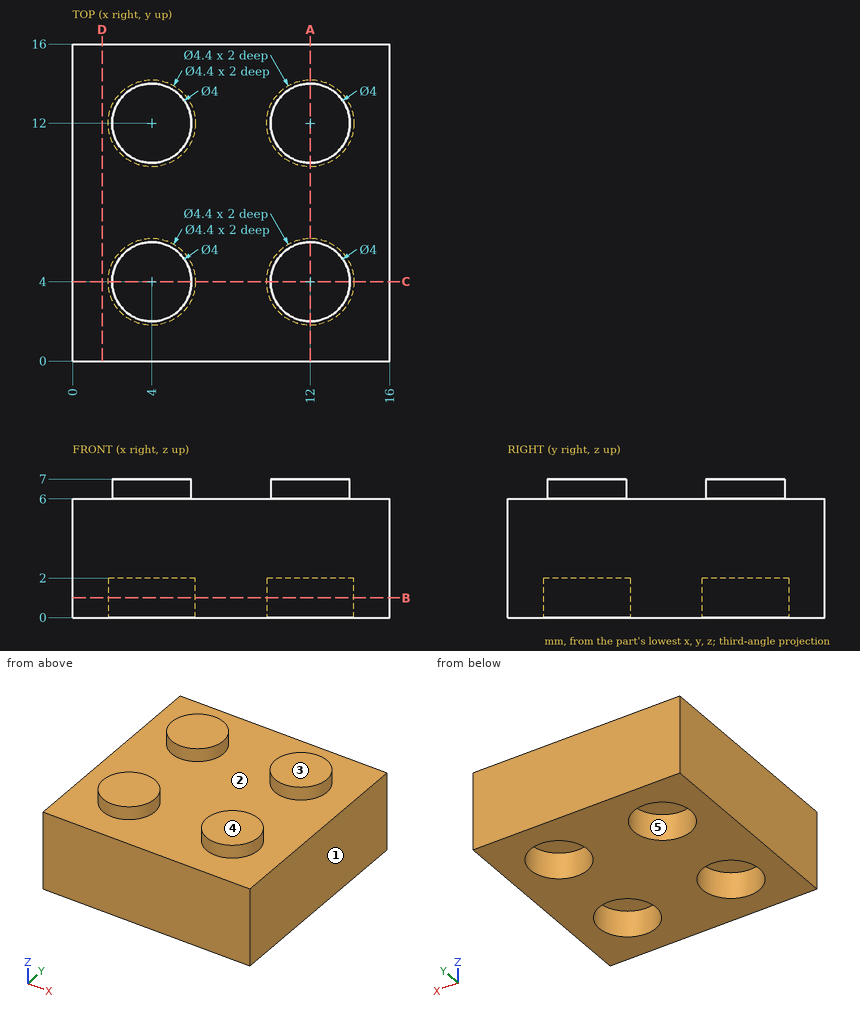
Input: dimensioned drawing with shaded views. Units: mm. Origin: part minimum x, y, z. A direction names the side the tool comes from. Coordinates: 2 decimals unless noted, no trailing zeros. Loops run counter-clockwise (first coordinate to the right, second up) from the corner with the lowest first, then second, coordinate; pieces in that order, holes last. Notation, with made-up numbers: M -30.5,-22.5 L -24.5,-22.5 A32 cw -24.5,14.5 Z; hole C 1,88 d9. An arc over 180 degrees is marked long. One line per item, written item: value.
(1) Section B-B (z = 1). Output: boundary loops of the cut face in (x, y).
Filled in:
outline: M 0,0 L 16,0 L 16,16 L 0,16 Z; hole C 4,4 d4.4; hole C 4,12 d4.4; hole C 12,4 d4.4; hole C 12,12 d4.4
(2) Section A-A (x = 12). Output: boundary loops of the cut face in (y, z), and give its area (3 significant figures).
Filled in:
outline: M 0,0 L 1.8,0 L 1.8,2 L 6.2,2 L 6.2,0 L 9.8,0 L 9.8,2 L 14.2,2 L 14.2,0 L 16,0 L 16,6 L 14,6 L 14,7 L 10,7 L 10,6 L 6,6 L 6,7 L 2,7 L 2,6 L 0,6 Z
area: 86.4 mm^2
(3) Pin query (flat end, axial travel): pin 1 (2.5 mm diameter, centred on x = 12, y = 12, fed in from -Z). Return the tip coordinate at first contact, or that it passes through.
Filled in:
pin 1: z = 2
(4) Pull-direction query (X, two-part tool) for the marked faces 1, 2 and 3; classes: +X half, -X half, draft (parallel to the pull), parting line (faces both ways), or undercut.
Filled in:
face 1: +X half
face 2: undercut
face 3: draft
(5) Reachability of the marked faces 4 and 5 from +Z, -Z, +X, -X, +Y, -Y: full face, straight path, thin tool, end or side. Return the list, or none.
Filled in:
face 4: +Z, +X, -X, +Y, -Y
face 5: -Z
(6) Section D-D (x = 1.5). Output: boundary loops of the cut face in (y, z).
Filled in:
outline: M 0,0 L 16,0 L 16,6 L 0,6 Z
(7) Line query: line 1 along X through (y, z) = (12, 1.2); line 2 along Z through (x, y) = (15.25, 6.75). Output: solid intervals per line, ascending. Write a range as from..to.
Filled in:
line 1: 0..1.8, 6.2..9.8, 14.2..16
line 2: 0..6
